Input: part model. Units: mm. Frame: model coordinates. Coordinates: 2 decimals unless noted, no trailing zeros. Loops run counter-clockwise (first coordinate to the right, second up) from the corner with the lowest first, then second, coordinate; pieces in that order, holes last.
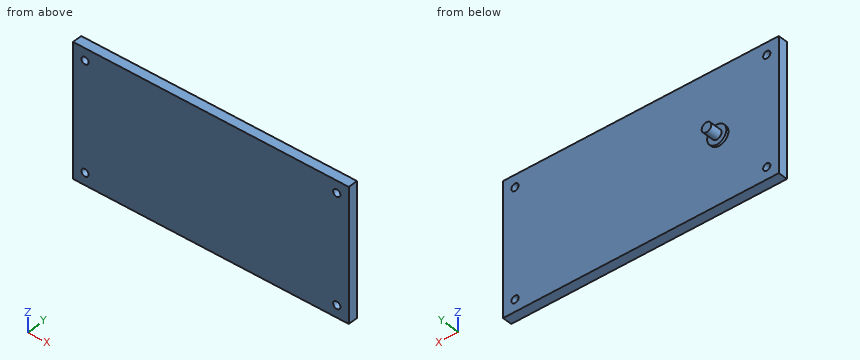
```python
from build123d import *

# Parameters (mm, degrees)
SKETCH_1_W          = 230
SKETCH_1_H          = 110
EXTRUDE_1_DEPTH     = 8
SKETCH_2_R          = 8
EXTRUDE_2_DEPTH     = 2
SKETCH_3_R          = 4
EXTRUDE_3_DEPTH     = 10
SKETCH_4_R          = 3
CUT_EXTRUDE_1_DEPTH = 129.039056541


with BuildPart() as part:
    # 草图1 → 凸台-拉伸1 (new body)
    with BuildSketch(Plane(origin=(0, 0, 0), x_dir=(1, 0, 0), z_dir=(0, 1, 0))):
        Rectangle(SKETCH_1_W, SKETCH_1_H)
    extrude(amount=EXTRUDE_1_DEPTH)

    # 草图2 → 凸台-拉伸2 (add)
    with BuildSketch(Plane(origin=(0, 8, 0), x_dir=(1, 0, 0), z_dir=(0, 1, 0))):
        with Locations(Location((-65, 0, 0), (0, 0, 270))):
            Circle(SKETCH_2_R)
    extrude(amount=EXTRUDE_2_DEPTH)

    # 草图3 → 凸台-拉伸3 (add)
    with BuildSketch(Plane(origin=(0, 10, 0), x_dir=(1, 0, 0), z_dir=(0, 1, 0))):
        with Locations(Location((-65, 0, 0), (0, 0, 270))):
            Circle(SKETCH_3_R)
    extrude(amount=EXTRUDE_3_DEPTH)

    # 草图4 → 切除-拉伸1 (cut, through all)
    with BuildSketch(Plane(origin=(0, 8, 0), x_dir=(1, 0, 0), z_dir=(0, 1, 0))):
        with Locations(Location((-105, 45, 0), (0, 0, 270))):
            Circle(SKETCH_4_R)
        with Locations(Location((-105, -45, 0), (0, 0, 270))):
            Circle(SKETCH_4_R)
        with Locations(Location((105, 45, 0), (0, 0, 270))):
            Circle(SKETCH_4_R)
        with Locations(Location((105, -45, 0), (0, 0, 270))):
            Circle(SKETCH_4_R)
    extrude(amount=-CUT_EXTRUDE_1_DEPTH, mode=Mode.SUBTRACT)


solid = part.part
```
Item 1: Section query C-C (z = 0). Output: boundary loops of the cut face in (x, y).
Result:
outline: (-115, 0) - (115, 0) - (115, 8) - (-57, 8) - (-57, 10) - (-61, 10) - (-61, 20) - (-69, 20) - (-69, 10) - (-73, 10) - (-73, 8) - (-115, 8) - close
Item 2: Section query B-B (x = -105). Output: boundary loops of the cut face in (y, z), then the cut area to 3 significant figures.
Result:
outline: (0, -55) - (8, -55) - (8, -48) - (0, -48) - close; (0, -42) - (8, -42) - (8, 42) - (0, 42) - close; (0, 48) - (8, 48) - (8, 55) - (0, 55) - close
area: 784 mm2
Item 3: Line query: L1, parallel to X at y = 6, z = 45; L2, parallel to X at y = 2.75, z = -47; L3, parallel to Y at x = -47.5, z = 4.5. Output: solid intervals per line, ascending.
Result:
L1: x = -115 to -108, -102 to 102, 108 to 115
L2: x = -115 to -107.24, -102.76 to 102.76, 107.24 to 115
L3: y = 0 to 8
Item 4: Section query A-A (z = 45). Output: boundary loops of the cut face in (x, y), then the cut area to 3 significant figures.
Result:
outline: (-115, 0) - (-108, 0) - (-108, 8) - (-115, 8) - close; (-102, 0) - (102, 0) - (102, 8) - (-102, 8) - close; (108, 0) - (115, 0) - (115, 8) - (108, 8) - close
area: 1,740 mm2
Item 5: Section query D-D (y = 13.75). Output: boundary loops of the cut face in (x, z).
Result:
outline: circle Ø8 at (-65, 0)
Item 6: Contact query for flat-ended pins moving along their axis: P1, Ø6, axis at y = 17.5, z = 6, coming from the +X side; P2, Ø9.5, axis at x = -105, z = -45, coming from the +Y side. Output: stop coordinate, or through.
Result:
P1: stops at x = -62.35
P2: stops at y = 8
